Design review of the part built by this model. Coordinates are the model's own, in mm. A direction names the side the tool comes from. Coordinates: 2 decimals unless noted, no trailing zeros. Loops run counter-clockwise (first coordinate to the right, second up) from the corner with the lowest first, then second, coordinate; pieces in that order, holes last. Notation, with made-up numbers: (18.5, 81) -> (60.5, 81) arc R18 cw to (60.5, 97) -> close; hole circle Ø6 at (53, 37). An arc over 180 degrees is marked (long way). Use one line per item in the form item = value. Start each with the question number.
1. Consider section D-D (y = -7.5). State the section outline as (x, z) points, then the cut area to 3 significant figures.
2. Consider section C-C (z = -52.5). State the section outline as (x, y) points, then the cut area to 3 significant figures.
3. Consider section A-A (x = 0). State the section outline as (y, z) points, then the cut area to 3 significant figures.
4. For pin 1 (1 mm diameter, centred on y = -0.5, z = -26, fed in from -X); pin 2 (6 mm diameter, centred on y = 4.5, z = -37, fed in from +X); pin 3 (3 mm diameter, centred on y = 3.5, z = -65, fed in from +X); pin 4 (1.5 mm diameter, centred on x = 1.5, y = -5.5, fed in from +Z), all flat-tipped, find the tip position at first contact; note any pin that passes through.
5. Machinability: for faces 1 (the face through (-3.32, -3.04, -42.98)), 2 (the face through (9.5, 0, -3)), which of the approach directions +Z, -Z, +X, -X, +Y, -Y give a long, thin tool a straight path to every point of the face, cutting with its end or side? Answer none if there is none.
6. Wall thickness on line 1 (Z direction, x = 8.75, y = -7); line 2 (Y direction, x = -0.25, z = -58.5); line 3 (Y direction, x = -4, z = -71): over which ranges is each line inside the solid? List them lowest first. Write a range as from..to.
from build123d import *

# Parameters (mm, degrees)
SKETCH1_W           = 19
SKETCH1_H           = 19
BOSS_EXTRUDE1_DEPTH = 6
SKETCH2_R           = 4.5
BOSS_EXTRUDE2_DEPTH = 76
CHAMFER1_SIZE       = 1


with BuildPart() as part:
    # Sketch1 → Boss-Extrude1 (new body)
    with BuildSketch(Plane.XY):
        Rectangle(SKETCH1_W, SKETCH1_H)
    extrude(amount=-BOSS_EXTRUDE1_DEPTH)

    # Sketch2 → Boss-Extrude2 (add)
    with BuildSketch(Plane(origin=(0, 0, -6), x_dir=(-1, 0, 0), z_dir=(0, 0, -1))):
        with Locations(Location((0, 0, 0), (0, 0, 180))):  # turned: the seam where the file's is
            Circle(SKETCH2_R)
    extrude(amount=BOSS_EXTRUDE2_DEPTH)

    # Chamfer1
    chamfer1_edges = [part.edges().sort_by_distance(p)[0] for p in [
        (-4.5, 0, -82),
    ]]
    chamfer(chamfer1_edges, length=CHAMFER1_SIZE)


solid = part.part
Geometry check:
q1.outline = (-9.5, -6) -> (9.5, -6) -> (9.5, 0) -> (-9.5, 0) -> close
q1.area = 114 mm²
q2.outline = circle Ø9 at (0, 0)
q2.area = 63.6 mm²
q3.outline = (-9.5, -6) -> (-4.5, -6) -> (-4.5, -81) -> (-3.5, -82) -> (3.5, -82) -> (4.5, -81) -> (4.5, -6) -> (9.5, -6) -> (9.5, 0) -> (-9.5, 0) -> close
q3.area = 797 mm²
q4.pin_1 = -4.5
q4.pin_2 = 4.24
q4.pin_3 = 4.03
q4.pin_4 = 0
q5.face_1 = -Z
q5.face_2 = +Z, -Z, +X, +Y, -Y
q6.line_1 = -6..0
q6.line_2 = -4.49..4.49
q6.line_3 = -2.06..2.06
